The model under review builds one solid part; all positions refer to its coordinate system, in mm. A direction names the side the tool comes from. Round coordinates to 2 decimals unless told otherwise and drop trailing zeros. Order: outer loops, then holes, each group sorted by start corner. A loop starts at its lowest first (then second) coordinate and runs counter-clockwise, first axis right, second up. Notation, with made-up numbers: M 60,-28 L 111,-28 A34 cw 111,3 Z; hole C 2,16 d1. An arc over 180 degrees is marked long. Use a Markdown table: item, result. Add a question column.
1. To check wall thickness, follow probe 1 along Y at (x, z) = (-16.3, -8.95); probe 2 along Y at (x, z) = (-16.3, -10.95); probe 3 along Z at (x, y) = (-14.75, 34.5). State the ranges of each line that lie inside material, in increasing order.
2. For faces 1 (the flat face through (-16, 20, -7.4)), 2 (the cylindrical face through (-15.65, 12.07, -11.82)), 3 (the flat face through (-19.3, 20, -1)), 4 (the cylindrical face through (-14.7, 25.07, -8.87)), 5 (the cylindrical face through (-20.7, 20.28, -12.73)), list the 3-axis set-ups (+Z, -Z, +X, -X, +Y, -Y) from which the entire face can be reached by the end or side of a thin tool; tool diameter is ignored.
3. Consider section B-B on y = 5. Count the separate pieces of the cut face and the enclosed holes in it, then the cut area to 3 significant figures.
4. The part is to be moulded in two halves that separate along X. For faces 6 (the cylindrical face through (-13.9, 3.2, -11.8)), 7 (the flat face through (-21.3, 20, -3)), 8 (the flat face through (-13, 40, -8)), say which applies: +X half, -X half, draft (parallel to the pull), parting line (faces both ways), or undercut.
5. Insertion check: P1, Ø5, axis at x = -16.3, y = 25, coming from the -Z side; P2, Ø2.5, axis at x = -16.3, y = 5, coming from the +Z side; P3, Ø1.2, axis at y = 20.5, z = -0.5, coming from the +X side; P4, Ø5, axis at x = -16, y = 11.5, coming from the +Z side. Each pin has a flat end and moves straight along its axis. Give the tip position at first contact, or say it passes through.
6. Consider section C-C on z = -1.25. State the section outline as (x, y) points.
7. Consider section A-A on x = -12.25. State the section outline as (y, z) points.
8. Consider section D-D on y = 11. State the section outline as (x, z) points.
Autodesk Inventor part; units mm, degrees
ref_plane "YZ Plane" through (0, 0, 0) normal (1, 0, 0) x (0, 1, 0)
ref_plane "XZ Plane" through (0, 0, 0) normal (0, 1, 0) x (-1, 0, 0)
ref_plane "XY Plane" through (0, 0, 0) normal (0, 0, 1) x (1, 0, 0)
sketch "Sketch1" plane through (0, 0, 0) normal (0, 1, 0) x (-1, 0, 0)
  line L0 (0, 0) -> (21.3, 0)
  line L1 (21.3, 0) -> (21.3, -13.3)
  line L2 (21.3, -13.3) -> (0, -13.3)
  line L3 (0, -13.3) -> (0, 0)
  dimension "d0" = 21.3
  dimension "d1" = 13.3
extrude "Extrusion1" add sketch "Sketch1" along normal blind 40
sketch "Sketch2" plane through (0, 40, 0) normal (0, 1, 0) x (1, 0, 0)
  circle A0 centre (-6.65, 6.65) radius 4.65
  line L0 (0, 0) -> (0, 13.3)
  line L1 (-21.3, 0) -> (0, 0)
  dimension "d4" = 9.3
  dimension "d5" = 6.65
  dimension "d6" = 6.65
extrude "Extrusion2" cut sketch "Sketch2" against normal through all
sketch "Sketch3" plane through (0, 40, 0) normal (0, 1, 0) x (1, 0, 0)
  line L0 (-21.3, 5.9) -> (-9.3, 5.9)
  line L1 (-9.3, 5.9) -> (-9.3, 7.4)
  line L2 (-9.3, 7.4) -> (-21.3, 7.4)
  line L3 (-21.3, 7.4) -> (-21.3, 5.9)
  line L4 (0, 13.3) -> (-21.3, 13.3)
  line L5 (-21.3, 13.3) -> (-21.3, 0)
  point P0 (0, 0)
  dimension "d9" = 1.5
  dimension "d10" = 5.9
  dimension "d11" = 12
extrude "Extrusion3" cut sketch "Sketch3" against normal through all
sketch "Sketch4" plane through (0, 40, 0) normal (0, 1, 0) x (1, 0, 0)
  line L0 (-19.3, 0) -> (-13.3, 0)
  line L1 (-13.3, 0) -> (-13.3, 2.5)
  line L2 (-13.3, 2.5) -> (-19.3, 2.5)
  line L3 (-19.3, 2.5) -> (-19.3, 0)
  line L4 (-21.3, 5.9) -> (-21.3, 0)
  line L5 (-21.3, 0) -> (0, 0)
  dimension "d14" = 2.5
  dimension "d15" = 6
  dimension "d16" = 2
extrude "Extrusion4" cut sketch "Sketch4" against normal through all
sketch "Sketch5" plane through (0, 0, -13.3) normal (0, 0, -1) x (-1, 0, 0)
  circle A0 centre (16.3, 35) radius 1.6
  line L0 (21.3, 0) -> (21.3, 40)
  line L1 (0, 40) -> (21.3, 40)
  point P0 (0, 0)
  dimension "d19" = 3.2
  dimension "d20" = 5
  dimension "d21" = 5
extrude "Extrusion5" cut sketch "Sketch5" against normal through all
pattern_linear "Rectangular Pattern1" count 4 spacing 10 along (0, -1, 0) of "Extrusion5"
sketch "Sketch6" plane through (0, 0, -13.3) normal (0, 0, -1) x (-1, 0, 0)
  line L0 (11.2391, 0) -> (11.2391, 40)
  circle A0 centre (16.3, 35) radius 3
  line L1 (21.3, 0) -> (21.3, 40)
  line L2 (0, 40) -> (21.3, 40)
  point P0 (0, 0)
  dimension "d27" = 6
  dimension "d28" = 5
  dimension "d29" = 5
extrude "Extrusion6" cut sketch "Sketch6" against normal blind 3
pattern_linear "Rectangular Pattern2" count 4 spacing 10 along (0, -1, 0) of "Extrusion6"
fillet "Fillet1" radius 2 3 edges at (0, 20, -13.3) (-21.3, 20, -13.3) (0, 20, 0)
equation "\"d6\" = d5"
properties part number "ADAPTATEUR"
Answer block:
| question | item | result |
|---|---|---|
| 1 | probe 1 | 0 to 3.4, 6.6 to 13.4, 16.6 to 23.4, 26.6 to 33.4, 36.6 to 40 |
| 1 | probe 2 | 0 to 2, 8 to 12, 18 to 22, 28 to 32, 38 to 40 |
| 1 | probe 3 | -10.3 to -7.4, -5.9 to -2.5 |
| 2 | face 1 | -X, +Y, -Y |
| 2 | face 2 | -Z |
| 2 | face 3 | +Z, +Y, -Y |
| 2 | face 4 | +Z, -Z |
| 2 | face 5 | -Z, -X, +Y, -Y |
| 3 | separate pieces | 3 |
| 3 | enclosed holes | 0 |
| 3 | area | 145 mm^2 |
| 4 | face 6 | undercut |
| 4 | face 7 | -X half |
| 4 | face 8 | draft |
| 5 | P1 | z = -10.3 |
| 5 | P2 | through |
| 5 | P3 | x = -0.21 |
| 5 | P4 | z = -2.5 |
| 6 | outline | M -21.3,0 L -19.3,0 L -19.3,40 L -21.3,40 Z; M -13.3,0 L -0.15,0 L -0.15,40 L -13.3,40 Z |
| 7 | outline | M 0,-13.3 L 40,-13.3 L 40,-7.4 L 0,-7.4 Z; M 0,-5.9 L 40,-5.9 L 40,0 L 0,0 Z |
| 8 | outline | M -21.3,-11.3 A2 ccw -19.3,-13.3 L -2,-13.3 A2 ccw 0,-11.3 L 0,-2 A2 ccw -2,0 L -13.3,0 L -13.3,-2.5 L -19.3,-2.5 L -19.3,0 L -21.3,0 L -21.3,-5.9 L -11.24,-5.9 A4.65 cw long -11.24,-7.4 L -21.3,-7.4 Z |
